Build history of the part. All positions in model axes, mm. Face numbers are marked on the shaded views. A direction names the side the tool comes from. Round coordinates to 2 decimals unless told otherwise and drop trailing zeros. Loops run counter-clockwise (first coordinate to the right, second up) from the corner with the lowest first, then second, coordinate; pieces in that order, holes last. Notation, with made-up numbers: M 28.5,30.25 L 55.5,30.25 A29 ccw 55.5,62.25 Z; hole C -7,-16 d1. An arc over 180 degrees is marked long. One line per item, written item: value.
```python
from build123d import *

# Parameters (mm, degrees)
BOSS_EXTRUDE1_DEPTH = 2


with BuildPart() as part:
    # Sketch1 → Revolve1 (revolve)
    with BuildSketch(Plane(origin=(0, 0, 0), x_dir=(1, 0, 0), z_dir=(0, 1, 0))):
        Polygon((-1.55, 0), (-6, 0), (-6, 2), (-3.75, 2), (-3.75, 4), (-6, 8.067249704), (-6, 11.5), (-5, 11.5), (-5, 9), (-2.688359629, 9), (-2.688359629, 7.5), (-1.55, 7.5), align=None)
    revolve(axis=Axis((0, 0, -14.260315956), (0, 0, 1)))

    # Sketch2 → Boss-Extrude1 (add)
    with BuildSketch(Plane.XY):
        with BuildLine():
            Line((-8.366600265, 1.5), (-5.809475019, 1.5))
            ThreePointArc((-5.809475019, 1.5), (-6, 0), (-5.809475019, -1.5))
            Line((-5.809475019, -1.5), (-8.366600265, -1.5))
            ThreePointArc((-8.366600265, -1.5), (-8.5, 0), (-8.366600265, 1.5))
        make_face()
        with BuildLine():
            Line((1.5, 8.366600265), (1.5, 5.809475019))
            ThreePointArc((1.5, 5.809475019), (0, 6), (-1.5, 5.809475019))
            Line((-1.5, 5.809475019), (-1.5, 8.366600265))
            ThreePointArc((-1.5, 8.366600265), (0, 8.5), (1.5, 8.366600265))
        make_face()
        with BuildLine():
            Line((8.366600265, -1.5), (5.809475019, -1.5))
            ThreePointArc((5.809475019, -1.5), (6, 0), (5.809475019, 1.5))
            Line((5.809475019, 1.5), (8.366600265, 1.5))
            ThreePointArc((8.366600265, 1.5), (8.5, 0), (8.366600265, -1.5))
        make_face()
        with BuildLine():
            Line((-1.5, -8.366600265), (-1.5, -5.809475019))
            ThreePointArc((-1.5, -5.809475019), (0, -6), (1.5, -5.809475019))
            Line((1.5, -5.809475019), (1.5, -8.366600265))
            ThreePointArc((1.5, -8.366600265), (0, -8.5), (-1.5, -8.366600265))
        make_face()
    extrude(amount=-BOSS_EXTRUDE1_DEPTH)


solid = part.part
```
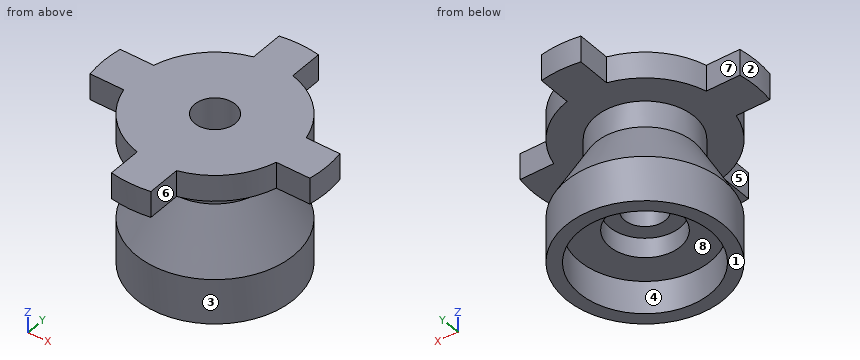
Item 1: Wall check: line 1 along X through (y, z) = (0, -8.1); line 2 along Y through (x, z) = (0, -3). Give the ranges that are in metal, low to high.
Check values:
line 1: x = -6 to -2.69, 2.69 to 6
line 2: y = -3.75 to -1.55, 1.55 to 3.75
Item 2: Drop flat-ended pins along their axis: P1, Ø0.6, axis at x = -7, z = -1, coming from the +Y side; P2, Ø2, axis at x = -4, z = -5.5, coming from the +Y side; P3, Ø1.6, axis at y = -7, z = -1.5, coming from the -X side. Give the stop position or say it passes through.
Check values:
P1: stops at y = 1.5
P2: stops at y = 3.73
P3: stops at x = -1.5
Item 3: Slice it at D-D, the plane y = -6.5. Give the cut face in (x, z), and give its area (3 significant figures).
Check values:
outline: M -1.5,-2 L 1.5,-2 L 1.5,0 L -1.5,0 Z
area: 6.00 mm2
Item 4: Slice it at C-C, the plane z = -10. Give the cut face in (x, y), and give its area (3 significant figures).
Check values:
outline: C 0,0 d12; hole C 0,0 d10
area: 34.6 mm2
Item 5: Pull direction X, two halves, no side cores. Call the marked faces 1, 2, 3 and 4: pulls with the +X half, pulls with the -X half, needs draft (parallel to the pull), parting line crosses it, or undercut.
Check values:
face 1: needs draft
face 2: pulls with the -X half
face 3: parting line crosses it
face 4: undercut
Item 6: Which spindle directions (+Z, -Z, +X, -X, +Y, -Y) get a long thin tool onto all of the face, cutting with end or side? Do the marked faces 5, 6, 7 and 8. Say none if no direction does.
Check values:
face 5: +Z, -Z, -X, -Y
face 6: +Z, -Z, +X, -Y
face 7: +Z, -Z, -X, +Y
face 8: -Z
Item 7: Slice it at A-A, the plane y = 0. Give the cut face in (x, z), and give its area (3 significant figures).
Check values:
outline: M -8.5,-2 L -3.75,-2 L -3.75,-4 L -6,-8.07 L -6,-11.5 L -5,-11.5 L -5,-9 L -2.69,-9 L -2.69,-7.5 L -1.55,-7.5 L -1.55,0 L -8.5,0 Z; M 1.55,-7.5 L 2.69,-7.5 L 2.69,-9 L 5,-9 L 5,-11.5 L 6,-11.5 L 6,-8.07 L 3.75,-4 L 3.75,-2 L 8.5,-2 L 8.5,0 L 1.55,0 Z
area: 73.5 mm2
